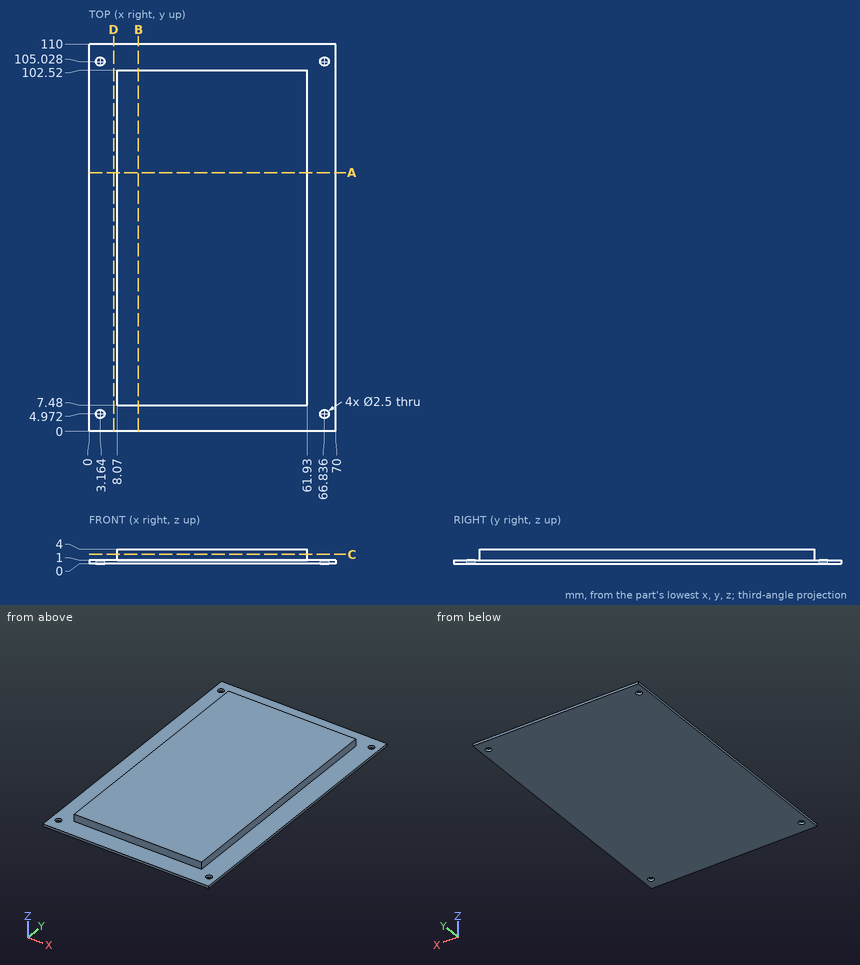
Answer from the drawing. Dimensions are ordinates in mm from the lowest x, y and z of the part. Round coordinates to 2 decimals unless told otherwise and drop trailing zeros. Loops run counter-clockwise (first coordinate to the right, second up) from the corner with the lowest first, then second, coordinate; pieces in that order, holes last. Notation, with made-up numbers: (-12, 87.25) - (-6, 87.25) arc R18 cw to (-6, 109.25) - close; hole circle Ø7 at (-37.75, 1.5). An arc over 180 degrees is marked (long way). One line per item, written item: value.
Q1. Find section B-B on x = 14. Give the vertices of the cut face in (y, z), and give its area (3 significant figures).
Check values:
outline: (0, 0) - (110, 0) - (110, 1) - (102.52, 1) - (102.52, 4) - (7.48, 4) - (7.48, 1) - (0, 1) - close
area: 395 mm2
Q2. Find section C-C on z = 2.6. Give the vertices of the cut face in (x, y).
Check values:
outline: (8.07, 7.48) - (61.93, 7.48) - (61.93, 102.52) - (8.07, 102.52) - close
Q3. Find section A-A on y = 73.5. Give the vertices of the cut face in (x, z), and give its area (3 significant figures).
Check values:
outline: (0, 0) - (70, 0) - (70, 1) - (61.93, 1) - (61.93, 4) - (8.07, 4) - (8.07, 1) - (0, 1) - close
area: 232 mm2
Q4. Each of these flat-tipped pins is pushed along its axis until it touches: pin 1 Ø3 at (x, y) = (66.84, 105.03) entering from +Z; pin 2 Ø12 at (x, y) = (44.5, 60) entering from -Z; pin 3 Ø2 at (x, y) = (3.16, 105.03) entering from +Z; pin 4 Ø0.9 at (y, z) = (75.5, 2) entering from +X. Where does it stop, or does it pass through?
Check values:
pin 1: z = 1
pin 2: z = 0
pin 3: through
pin 4: x = 61.93
Q5. Find section D-D on x = 7. Give the vertices of the cut face in (y, z).
Check values:
outline: (0, 0) - (110, 0) - (110, 1) - (0, 1) - close
Q6. Straight lines are drawn through the part: probe 1 along X at (y, z) = (18.5, 1.5); probe 2 along Y at (x, z) = (37.5, 3.3); probe 3 along Z at (x, y) = (66.5, 29). For each, find the intervals that lie inside material, in ascending order.
Check values:
probe 1: 8.07 to 61.93
probe 2: 7.48 to 102.52
probe 3: 0 to 1
